Design review of the part built by this model. Coordinates are the model's own, in mm. Face numbers are marked on the shaded views. A direction names the side the tool comes from. Coordinates: 2 decimals unless noted, no trailing zeros. Write each loop counter-clockwise with the first axis right and the second up, starting at its lowest first coordinate (ties: lowest second). Pieces come first, ordered by that corner, then holes. Notation, with made-up numbers: (-24, 34.5) - (-12, 34.5) arc R28 cw to (-12, 52.5) - close; hole circle Ø7 at (16, 54). An arc over 180 degrees is marked (long way). Use a Markdown table: item, result.
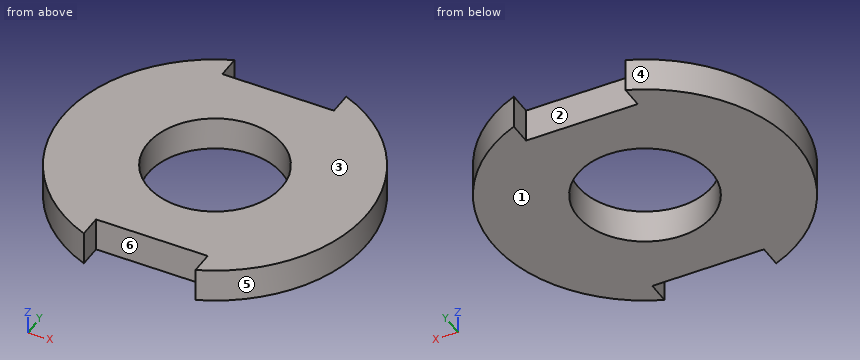
from build123d import *

# Parameters (mm, degrees)
SKETCH_1_R          = 13.6
SKETCH_1_R_2        = 6
EXTRUDE_1_DEPTH     = 3
SKETCH_2_W          = 10
SKETCH_2_H          = 6
CUT_EXTRUDE_1_DEPTH = 3


with BuildPart() as part:
    # 스케치1 → 보스-돌출1 (new body)
    with BuildSketch(Plane.XY):
        Circle(SKETCH_1_R)
        Circle(SKETCH_1_R_2, mode=Mode.SUBTRACT)
    extrude(amount=EXTRUDE_1_DEPTH)

    # 스케치2 → 컷-돌출1 (cut)
    with BuildSketch(Plane(origin=(0, 0, 0), x_dir=(-1, 0, 0), z_dir=(0, 0, -1))):
        with Locations((0, -13.6)):
            Rectangle(SKETCH_2_W, SKETCH_2_H)
        with Locations((0, 13.6)):
            Rectangle(SKETCH_2_W, SKETCH_2_H)
    extrude(amount=-CUT_EXTRUDE_1_DEPTH, mode=Mode.SUBTRACT)


solid = part.part
(1) For pin 1 (1 mm diameter, centred on y = 12, z = 2, fed in from -X); pin 2 (1 mm diameter, centred on y = -11, z = 1, fed in from +X); pin 3 (0.6 mm diameter, centred on y = 12, z = 1.5, fed in from +X), all flat-tipped, find the tip position at first contact; note any pin that passes through.
Determined:
| item | result |
|---|---|
| pin 1 | x = -7.26 |
| pin 2 | x = 8.64 |
| pin 3 | x = 6.93 |
(2) Draft analysis for pull direction X (two halves, no side actions). For the marked faces 3, 4, 5 and 6, state which applies: +X half, -X half, draft (parallel to the pull), parting line (faces both ways), or undercut.
Determined:
| item | result |
|---|---|
| face 3 | draft |
| face 4 | -X half |
| face 5 | +X half |
| face 6 | undercut |
(3) For L1, parallel to Y at x = 0, z = 1; L2, parallel to X at y = -2, z = 0.7; L3, parallel to Y at x = -4.5, z = 1.35, list the stretches that pass through material, from the lowest coordinate up. Write a range as from..to.
Determined:
| item | result |
|---|---|
| L1 | -10.6..-6, 6..10.6 |
| L2 | -13.45..-5.66, 5.66..13.45 |
| L3 | -10.6..-3.97, 3.97..10.6 |
(4) Take a section at B-B on x = 0. Write out the cut boundary in (y, z), and give its area (3 significant figures).
Determined:
| item | result |
|---|---|
| outline | (-10.6, 0) - (-6, 0) - (-6, 3) - (-10.6, 3) - close; (6, 0) - (10.6, 0) - (10.6, 3) - (6, 3) - close |
| area | 27.6 mm2 |
(5) Take a section at C-C on z = 1.25. Write out the cut boundary in (x, y), and give its area (3 significant figures).
Determined:
| item | result |
|---|---|
| outline | (-5, -12.65) - (-5, -10.6) - (5, -10.6) - (5, -12.65) arc R13.6 ccw to (5, 12.65) - (5, 10.6) - (-5, 10.6) - (-5, 12.65) arc R13.6 ccw to start; hole circle Ø12 at (0, 0) |
| area | 414 mm2 |
(6) Machinability: for the marked faces 1 and 2, which of the approach directions +Z, -Z, +X, -X, +Y, -Y give a long, thin tool a straight path to every point of the face, cutting with its end or side? Answer none if there is none.
Determined:
| item | result |
|---|---|
| face 1 | -Z, +X, -X, +Y, -Y |
| face 2 | +Z, -Z, +Y |
(7) Take a section at D-D on y = -7.25. Write out the cut boundary in (x, z), and give its area (3 significant figures).
Determined:
| item | result |
|---|---|
| outline | (-11.51, 0) - (11.51, 0) - (11.51, 3) - (-11.51, 3) - close |
| area | 69.0 mm2 |
(8) Take a section at A-A on y = 0. Write out the cut boundary in (x, z).
Determined:
| item | result |
|---|---|
| outline | (-13.6, 0) - (-6, 0) - (-6, 3) - (-13.6, 3) - close; (6, 0) - (13.6, 0) - (13.6, 3) - (6, 3) - close |
